from build123d import *

# Parameters (mm, degrees)
F0_W     = 20
F0_H     = 6
F1_DEPTH = 0.75
F3_DEPTH = 4.5
F4_R     = 1
F6_R     = 2.99999
F8_DEPTH = 3.5


# Not quite as in the source:
# - a fillet or chamfer is up to 0.001 mm smaller than in the source, because OpenCascade refuses the exact size


with BuildPart() as f1:
    # F0 (on Top) → F1 (new body)
    with BuildSketch(Plane.XY):
        with Locations((-4, 0)):
            Rectangle(F0_W, F0_H)
    extrude(amount=F1_DEPTH)

    # F2 (on face) → F3 (join)
    with BuildSketch(Plane.XY.offset(0.75)):
        with BuildLine():
            ThreePointArc((0, -3), (2.1213203436, -2.1213203436), (3, 0))
            ThreePointArc((3, 0), (2.1213203436, 2.1213203436), (0, 3))
            ThreePointArc((0, 3), (-3, 0), (0, -3))
        make_face()
    extrude(amount=F3_DEPTH)

    # F4 (on face) → F5 (revolve, cut)
    with BuildSketch(Plane.XY.offset(5.25)):
        Circle(F4_R)
    revolve(axis=Axis((-3, -2.9594153166, 5.25), (0, -1, 0)), mode=Mode.SUBTRACT)

    # F6 (radius 3 in the source; OpenCascade refuses exactly that, so slightly less here)
    f6_edges = [f1.edges().sort_by_distance(p)[0] for p in [
        (6, -3, 0.375),
        (6, 3, 0.375),
    ]]
    fillet(f6_edges, radius=F6_R)

    # F7 (on face) → F8 (join)
    with BuildSketch(Plane.XY.offset(0.75)):
        with BuildLine():
            Line((-2.5980762114, 1.5), (-14, 1.5))
            Line((-14, 1.5), (-14, 1.2))
            Line((-14, 1.2), (-2.749545417, 1.2))
            ThreePointArc((-2.749545417, 1.2), (-2.6780149869, 1.3521226757), (-2.5980762114, 1.5))
        make_face()
        with BuildLine():
            Line((-2.749545417, -1.2), (-14, -1.2))
            Line((-14, -1.2), (-14, -1.5))
            Line((-14, -1.5), (-2.5980762114, -1.5))
            ThreePointArc((-2.5980762114, -1.5), (-2.6780149869, -1.3521226757), (-2.749545417, -1.2))
        make_face()
    extrude(amount=F8_DEPTH)


solid = f1.part
Model file for the job. Use its own axes, mm. A direction names the side the tool comes from. Coordinates: 2 decimals unless noted, no trailing zeros. Order: outer loops, then holes, each group sorted by start corner. A loop starts at its lowest first (then second) coordinate and runs counter-clockwise, first axis right, second up. Notation, with made-up numbers: (6, 49) -> (60, 49) arc R16 cw to (60, 73) -> close; hole circle Ø8 at (70.5, -28). An arc over 180 degrees is marked (long way). Return JSON: item names as keys, results as strings. Group by question number.
Item 1: Pull direction Y, two halves, no side cores. Call faces 5 (the flat face through (-8, 1.5, 2)), 6 (the flat face through (-8, 0, 0.75)), 7 (the flat face through (-8, -1.5, 2)): pulls with the +Y half, pulls with the -Y half, needs draft (parallel to the pull), parting line crosses it, or undercut.
Item 2: Flat gauge pins, fed straight in: P1, Ø3, axis at x = -10.5, z = 2.5, coming from the +Y side; P2, Ø1.2, axis at x = -10, y = 2, coming from the +Z side; P3, Ø1, axis at y = -0.5, z = 3, coming from the +X side. Where does each tip first touch, or does it go through?
Item 3: Saw through at A-A on x = -8. Write the cut outline in (y, z).
Item 4: Wall check: line 1 along Y through (x, z) = (-9, 2.3); line 2 along Z through (x, y) = (4.5, -2.5); line 3 along Z through (x, y) = (-1.5, 0.25). Give the ranges that are in metal, low to high. Write a range as [from, to].
Item 5: Saw through at B-B on y = 1.75. Write the cut outline in (x, z), then the cut area to 3 significant figures.
Item 6: Tool access for faces 1 (the flat face through (4, 0, 0.75)), 2 (the flat face through (-9, -2, 0.75)), 3 (the flat face through (-8, -1.2, 2)), 4 (the flat face through (-7, 2, 0.75)): list every direction of +Z, -Z, +X, -X, +Y, -Y with a clear straight run to the whole face (end or side of a thin tool).
Values found:
{
 "1": {"face 5": "pulls with the +Y half", "face 6": "undercut", "face 7": "pulls with the -Y half"},
 "2": {"P1": "stops at y = 1.5", "P2": "stops at z = 4.25", "P3": "stops at x = 3"},
 "3": {"outline": "(-3, 0) -> (3, 0) -> (3, 0.75) -> (1.5, 0.75) -> (1.5, 4.25) -> (1.2, 4.25) -> (1.2, 0.75) -> (-1.2, 0.75) -> (-1.2, 4.25) -> (-1.5, 4.25) -> (-1.5, 0.75) -> (-3, 0.75) -> close"},
 "4": {"line 1": "y = [-1.5, -1.2], [1.2, 1.5]", "line 2": "z = [0, 0.75]", "line 3": "z = [0, 1.58], [3.88, 5.25]"},
 "5": {"outline": "(-14, 0) -> (5.44, 0) -> (5.44, 0.75) -> (2.44, 0.75) -> (2.44, 5.25) -> (-2.44, 5.25) -> (-2.44, 0.75) -> (-14, 0.75) -> close", "area": "36.5 mm2"},
 "6": {"face 1": "+Z, +X", "face 2": "+Z, -X, -Y", "face 3": "+Z, -X", "face 4": "+Z, -X, +Y"}
}
